Autodesk Inventor part; units mm, degrees
ref_plane "YZ Plane" through (0, 0, 0) normal (1, 0, 0) x (0, 1, 0)
ref_plane "XZ Plane" through (0, 0, 0) normal (0, 1, 0) x (-1, 0, 0)
ref_plane "XY Plane" through (0, 0, 0) normal (0, 0, 1) x (1, 0, 0)
sketch "Sketch1" plane through (0, 0, 0) normal (0, 0, 1) x (1, 0, 0)
  line L0 (-12.7, -25.4) -> (12.7, -25.4)
  line L1 (12.7, -25.4) -> (12.7, 25.4)
  line L2 (12.7, 25.4) -> (-12.7, 25.4)
  line L3 (-12.7, 25.4) -> (-12.7, -25.4)
  line L4 (-12.7, -25.4) -> (12.7, 25.4) construction
  line L5 (12.7, -25.4) -> (-12.7, 25.4) construction
  line L6 (-11.1125, 23.8125) -> (11.1125, 23.8125)
  line L7 (11.1125, 23.8125) -> (11.1125, -23.8125)
  line L8 (11.1125, -23.8125) -> (-11.1125, -23.8125)
  line L9 (-11.1125, -23.8125) -> (-11.1125, 23.8125)
  point P0 (0, 0)
  dimension "width" = 25.4
  dimension "height" = 50.8
  dimension "thickness" = 1.5875
extrude "Extrusion1" add sketch "Sketch1" along normal mid plane 254
sketch "Sketch2" plane through (-12.7, -25.4, 127) normal (-1, 0, 0) x (0, 0, 1)
  line L0 (-254, 0) -> (-254, 50.8) construction
  line L1 (-254, 50.8) -> (0, 50.8) construction
  line L2 (0, 50.8) -> (0, 0) construction
  line L3 (0, 0) -> (-254, 0) construction
  point P0 (-127, 25.4)
  point P1 (-241.3, 38.1)
  point P2 (-241.3, 25.4)
  point P3 (-241.3, 12.7)
  point P4 (-12.7, 38.1)
  point P5 (-12.7, 25.4)
  point P6 (-12.7, 12.7)
  point P7 (-254, 25.4)
  dimension "d5" = 12.7
  dimension "d6" = 12.7
  dimension "d7" = 12.7
  dimension "d8" = 12.7
hole "Block Mount Holes" at (-12.7, 12.7, -114.3) at (-12.7, 0, -114.3) at (-12.7, -12.7, -114.3) at (-12.7, 12.7, 114.3) at (-12.7, 0, 114.3) at (-12.7, -12.7, 114.3) direction (1, 0, 0) diameter 5.1054 end through all
sketch "Sketch4" plane through (-12.7, 25.4, 127) normal (0, 1, 0) x (1, 0, 0)
  line L0 (0, 254) -> (25.4, 254)
  line L1 (12.7, 190.5) -> (12.7, 63.5) construction
  point P0 (12.7, 127)
  point P1 (12.7, 254)
  point P2 (12.7, 203.2)
  point P3 (12.7, 50.8)
  point P4 (12.7, 127)
  dimension "d61" = 12.7
  dimension "d65" = 127
  dimension "d66" = 12.7
hole "Hole3" at (0, 25.4, 63.5) at (0, 25.4, -63.5) at (0, 25.4, -76.2) at (0, 25.4, 76.2) direction (0, -1, 0) diameter 5.1054 end through all
sketch "Sketch8" plane through (-12.7, 25.4, 127) normal (0, 1, 0) x (1, 0, 0)
  circle A0 centre (12.7, 203.2) radius 2.5527 construction
  circle A1 centre (12.7, 63.5) radius 2.5527 construction
  circle A2 centre (12.7, 190.5) radius 2.5527 construction
  circle A3 centre (12.7, 50.8) radius 2.5527 construction
  line L0 (0, 254) -> (25.4, 254) construction
  line L1 (25.4, 254) -> (25.4, 0) construction
  line L2 (25.4, 0) -> (0, 0) construction
  line L3 (0, 0) -> (0, 254) construction
  point P0 (12.7, 127)
  point P1 (12.7, 127)
  point P2 (12.7, 101.6)
  point P3 (9.9314, 152.4)
  dimension "d67" = 25.4
  dimension "d68" = 25.4
hole "Hole5" at (0, 25.4, 0) at (0, 25.4, 25.4) direction (0, -1, 0) diameter 5.1054 end through all
sketch "Sketch9" plane through (-12.7, 25.4, 127) normal (0, 1, 0) x (1, 0, 0)
  line L0 (0, 254) -> (25.4, 254)
  line L1 (25.4, 0) -> (0, 0)
  point P0 (12.7, 127)
  point P1 (12.7, 12.7)
  point P2 (12.7, 241.3)
  point P3 (12.7, 254)
  point P4 (12.7, 254)
  point P5 (12.7, 0)
  dimension "d79" = 12.7
  dimension "d80" = 12.7
hole "Hole6" at (0, 25.4, 114.3) at (0, 25.4, -114.3) direction (0, -1, 0) diameter 5.1054 end through all
sketch "Sketch10" plane through (12.7, -25.4, 127) normal (1, 0, 0) x (0, 0, -1)
  line L0 (254, 50.8) -> (254, 0)
  line L1 (184.15, 40.3225) -> (184.15, 10.4775) construction
  point P0 (127, 25.4)
  point P1 (184.15, 25.4)
  point P2 (254, 25.4)
  point P3 (149.225, 25.4)
  point P4 (254, 25.4)
  dimension "d88" = 69.85
  dimension "d89" = 29.845
  dimension "d97" = 104.775
hole "Hole8" at (12.7, 0, -22.225) direction (-1, 0, 0) diameter 5.1054 end through all
sketch "Sketch11" plane through (12.7, -25.4, 127) normal (1, 0, 0) x (0, 0, -1)
  line L0 (76.2, 31.75) -> (76.2, 19.05) construction
  line L1 (0, 0) -> (0, 50.8) construction
  point P0 (127, 25.4)
  point P1 (76.2, 25.4)
  point P2 (0, 25.4)
  dimension "d105" = 76.2
  dimension "d106" = 12.7
hole "Hole9" at (12.7, 6.35, 50.8) at (12.7, -6.35, 50.8) direction (-1, 0, 0) diameter 5.1054 end through all
mirror "Mirror1" about plane through (0, 0, 0) normal (0, 0, 1) of "Hole9"
sketch "Sketch13" plane through (12.7, -25.4, 127) normal (1, 0, 0) x (0, 0, -1)
  circle A0 centre (177.8, 19.05) radius 2.5527
  circle A1 centre (177.8, 31.75) radius 2.5527
  circle A2 centre (76.2, 31.75) radius 2.5527
  circle A3 centre (76.2, 19.05) radius 2.5527
  circle A4 centre (149.225, 25.4) radius 2.5527
  circle A5 centre (12.7, 25.4) radius 2.5527
  circle A6 centre (241.3, 12.7) radius 2.5527
  circle A7 centre (241.3, 38.1) radius 2.5527
  circle A8 centre (241.3, 25.4) radius 2.5527
  circle A9 centre (12.7, 38.1) radius 2.5527
  circle A10 centre (12.7, 12.7) radius 2.5527
  line L0 (254, 50.8) -> (254, 0)
  line L1 (254, 0) -> (0, 0)
  line L2 (0, 0) -> (0, 50.8)
  line L3 (0, 50.8) -> (254, 50.8)
  circle A11 centre (149.225, 25.4) radius 2.5527
  circle A12 centre (149.225, 25.4) radius 6.35
  point P0 (127, 25.4)
  dimension "d117" = 12.7
extrude "Extrusion5" cut sketch "Sketch13" against normal up to surface (1.5875 mm away) contours A12
sketch "Sketch14" plane through (12.7, -25.4, 127) normal (1, 0, 0) x (0, 0, -1)
  line L0 (227.3376, 44.45) -> (227.3376, 6.35) construction
  line L1 (254, 50.8) -> (254, 0) construction
  line L2 (31.75, 44.45) -> (31.75, 6.35) construction
  line L3 (0, 0) -> (0, 50.8) construction
  point P0 (127, 25.4)
  point P1 (227.3376, 25.4)
  point P2 (254, 25.4)
  point P3 (31.75, 25.4)
  point P4 (0, 25.4)
  dimension "d120" = 38.1
  dimension "d121" = 26.6624
  dimension "d129" = 38.1
  dimension "d130" = 31.75
hole "Hole10" at (12.7, 19.05, -100.3376) at (12.7, -19.05, -100.3376) at (12.7, 19.05, 95.25) at (12.7, -19.05, 95.25) direction (-1, 0, 0) diameter 5.1054 end through all
properties part number "EL2-C-005" material "Aluminum 6061"
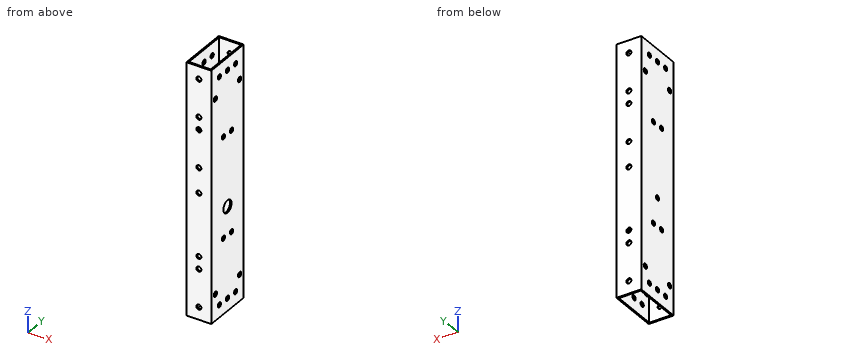
Check sheet for the modelled part. Datum: model origin and axes. Units: mm. Give positions to 0.01 mm unless a question says otherwise; leave off trailing zeros. Loops run counter-clockwise (first coordinate to the right, second up) from the corner with the lowest first, then second, coordinate; pieces in that order, holes last. Notation, with made-up numbers: M 21,64 L 38,64 A20 cw 38,73 Z; hole C 46,54 d2. An arc over 180 degrees is marked long. Answer as a JSON object with one key per item and string values. Group by question number.
Q1. Material ranges on line 1 along Y through (x, z) = (-11.5, 50.8); line 2 along Y through (x, z) = (6, -109.5); line 3 along Z through (x, y) = (-11.45, -19.05), recorded low to high. Write a range as [from, to].
Q2. Cross-section at D-D on z = -114.3. Give the number of separate pieces and of enclosed holes in the cut face, then the cut area to 3 significant figures.
Q3. Cross-section at C-C on z = 35. Record the cut outline in (x, y), then the cut area to 3 significant figures.
Q4. Cross-section at A-A on z = 76.2. Record the cut outline in (x, y), then the cut area to 3 significant figures.
Q5. Cross-section at B-B on y = -19.05. Record the cut outline in (x, z), then the cut area to 3 significant figures.
Evaluation:
{
 "1": {"line 1": "y = [-25.4, -8.9], [-3.8, 3.8], [8.9, 25.4]", "line 2": "y = [-25.4, -23.81], [23.81, 25.4]", "line 3": "z = [-127, -102.89], [-97.78, 92.7], [97.8, 127]"},
 "2": {"separate pieces": "8", "enclosed holes": "0", "area": "167 mm2"},
 "3": {"outline": "M -12.7,-25.4 L 12.7,-25.4 L 12.7,25.4 L -12.7,25.4 Z; hole M -11.11,-23.81 L 11.11,-23.81 L 11.11,23.81 L -11.11,23.81 Z", "area": "232 mm2"},
 "4": {"outline": "M -12.7,-25.4 L -2.55,-25.4 L -2.55,-23.81 L -11.11,-23.81 L -11.11,23.81 L -2.55,23.81 L -2.55,25.4 L -12.7,25.4 Z; M 2.55,-25.4 L 12.7,-25.4 L 12.7,25.4 L 2.55,25.4 L 2.55,23.81 L 11.11,23.81 L 11.11,-23.81 L 2.55,-23.81 Z", "area": "216 mm2"},
 "5": {"outline": "M -12.7,-127 L -11.11,-127 L -11.11,-102.89 L -12.7,-102.89 Z; M -12.7,-97.78 L -11.11,-97.78 L -11.11,92.7 L -12.7,92.7 Z; M -12.7,97.8 L -11.11,97.8 L -11.11,127 L -12.7,127 Z; M 11.11,-127 L 12.7,-127 L 12.7,-102.89 L 11.11,-102.89 Z; M 11.11,-97.78 L 12.7,-97.78 L 12.7,92.7 L 11.11,92.7 Z; M 11.11,97.8 L 12.7,97.8 L 12.7,127 L 11.11,127 Z", "area": "774 mm2"}
}
